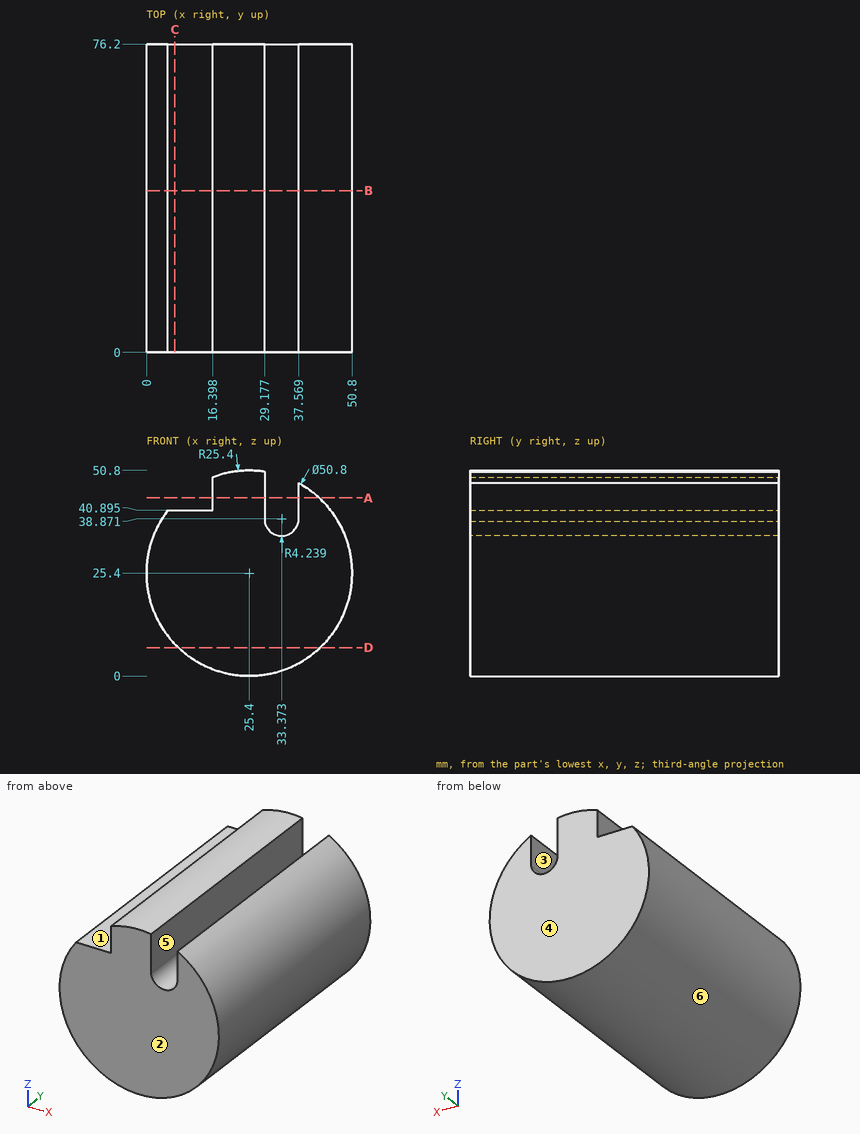
Check sheet for the drawn part. Datum: minimum x, y, z corner. Units: mm. A direction names the side the tool comes from. Round coordinates to 2 decimals unless told otherwise and drop trailing zeros. Write each loop counter-clockwise with the first axis right and the second up, starting at its lowest first coordinate (ties: lowest second). Pieces come first, ordered by that corner, then holes. Notation, with made-up numbers: (-24, 82) - (31, 82) arc R31 ccw to (31, 117) - close; hole circle Ø3 at (61.5, 64.25). An arc over 180 degrees is marked (long way). Return JSON: item names as keys, results as strings.
Q1. Draft check along X on the marked faces 4, 5 and 6. Enter one of: released by +X, released by -X, zero draft, split by the parting line, or undercut.
Returned:
{"face 4": "zero draft", "face 5": "undercut", "face 6": "split by the parting line"}
Q2. Cross-section at C-C (x = 7). Record the boundary of the cut face in (y, z) (1 decimal), then the cut area to 4 significant figures.
Returned:
{"outline": "(0, 7.9) - (76.2, 7.9) - (76.2, 40.9) - (0, 40.9) - close", "area": "2,515 mm²"}
Q3. Scan lines: L1, parallel to X at y = 23, z = 47 (1 decimal); L2, parallel to X at y = 29, z = 36 (1 decimal); L3, parallel to Z at x = 38.5, y = 22. Record each from-to range of solid material in increasing order. Write a range as from..to.
Returned:
{"L1": "x = 16.4..29.2, 37.6..38.8", "L2": "x = 2.3..30.3, 36.5..48.5", "L3": "z = 3.64..47.16"}
Q4. Cross-section at D-D (z = 7). Record the boundary of the cut face in (x, y), then the cut area to 3 significant figures.
Returned:
{"outline": "(7.89, 0) - (42.91, 0) - (42.91, 76.2) - (7.89, 76.2) - close", "area": "2,670 mm²"}
Q5. Access from +Z, -Z, +X, -X, +Y, -Y to the whole of each face (thin tool, end or side, straight path). Record for the marked faces 1, 2 and 3.
Returned:
{"face 1": "+Z, -X, +Y, -Y", "face 2": "+Z, -Z, +X, -X, -Y", "face 3": "+Z, +Y, -Y"}
Q6. Cross-section at A-A (z = 44). Record the boundary of the cut face in (x, y).
Returned:
{"outline": "(16.4, 0) - (29.18, 0) - (29.18, 76.2) - (16.4, 76.2) - close; (37.57, 0) - (42.7, 0) - (42.7, 76.2) - (37.57, 76.2) - close"}
Q7. Cross-section at B-B (y = 40). Record the boundary of the cut face in (x, z) (1 decimal), then the cut area to 3 significant figures.
Returned:
{"outline": "(5.3, 40.9) arc R25.4 ccw (long way) to (37.6, 47.7) - (37.6, 38.3) arc R4.2 cw to (29.2, 38.3) - (29.2, 50.5) arc R25.4 ccw to (16.4, 49.2) - (16.4, 40.9) - close", "area": "1,860 mm²"}
Q8. Depth check by flat-ended pin: P1, Ø10.5, axis at y = 49.5, z = 43, coming from the -X side (1 decimal); P2, Ø8, axis at y = 20, z = 16.5, coming from the -X side; P3, Ø12, axis at x = 30, y = 66, coming from the -Z side. Enter the tip coordinate at first touch or a pass-through.
Returned:
{"P1": "stops at x = 3.2", "P2": "stops at x = 0.48", "P3": "stops at z = 0"}
